Verification items for the finished model (mm, model axes). Round coordinates to 2 decimals unless told otherwise and drop trailing zeros. Loops run counter-clockwise (first coordinate to the right, second up) from the corner with the lowest first, then second, coordinate; pieces in that order, holes last. Notation, with made-up numbers: M 26.5,-38.5 L 63.5,-38.5 A21 cw 63.5,-27.5 Z; hole C -1.5,81.25 d5. An arc over 180 degrees is marked long. Write item = value, one per line. Start each with the question number.
Autodesk Inventor part; units mm, degrees
ref_plane "YZ Plane" through (0, 0, 0) normal (1, 0, 0) x (0, 1, 0)
ref_plane "XZ Plane" through (0, 0, 0) normal (0, 1, 0) x (-1, 0, 0)
ref_plane "XY Plane" through (0, 0, 0) normal (0, 0, 1) x (1, 0, 0)
ref_plane "Work Plane1" through (3, 4, -1) normal (0, 0, 1) x (0, -1, 0)
sketch "Sketch1" plane through (3, 4, -1) normal (0, 0, 1) x (0, -1, 0)
  line L0 (18.0177, 33.5) -> (5, 33.5)
  line L1 (5, 0) -> (5, 33.5)
  line L2 (5, 0) -> (89.75, 0)
  line L3 (89.75, 0) -> (89.75, 33.5)
  line L4 (5, 0) -> (60, 0)
  line L5 (5, -3) -> (5, 0)
  line L6 (4, -3) -> (60, -3)
  line L7 (60, 33.5) -> (60, 3.25)
  line L8 (60, -3) -> (60, 0)
  arc A0 (63.25, 0) -> (60, 3.25) centre (63.25, 3.25) ccw
  line L9 (88.5, 0) -> (183, 0)
  circle A1 centre (75.375, 15.375) radius 6.75
  line L10 (60, 0) -> (60, 33.5)
  circle A2 centre (32.5, 10.5) radius 5.5
  circle A3 centre (9, 4) radius 2.1
  circle A4 centre (9, 29.5) radius 2.1
  circle A5 centre (56.5, 3.5) radius 2.1
  spline S0 degree 2 poles (19.3669, 33.5) (18.6923, 33.3555) (18.0177, 33.5) knots 0 0 0 0.135703 0.135703 0.135703 weights 1 1.02375 1
  line L11 (89.75, 33.5) -> (85.2105, 33.5)
  spline S1 degree 2 poles (85.2105, 33.5) (84.25, 33.2071) (83.2895, 33.5) knots 0 0 0 0.194422 0.194422 0.194422 weights 1 1.05 1
  line L12 (83.2895, 33.5) -> (66.5855, 33.5)
  spline S2 degree 2 poles (66.5855, 33.5) (65.625, 33.2071) (64.6645, 33.5) knots 0 0 0 0.194422 0.194422 0.194422 weights 1 1.05 1
  line L13 (64.6645, 33.5) -> (47.1605, 33.5)
  spline S3 degree 2 poles (47.1605, 33.5) (46.2, 33.2071) (45.2395, 33.5) knots 0 0 0 0.194422 0.194422 0.194422 weights 1 1.05 1
  line L14 (45.2395, 33.5) -> (19.3669, 33.5)
  line L15 (63.25, 0) -> (88.5, 0)
  circle A6 centre (88.5, 3.25) radius 3.25
  line L16 (183, 0) -> (183, 4.5)
  line L17 (183, 4.5) -> (137.8889, 33.5)
  line L18 (137.8889, 33.5) -> (60, 33.5)
  point P0 (52, 0)
  point P1 (64.076, 0)
  point P2 (87.674, 0)
  point P3 (63.25, 3.25)
  point P4 (60, 3.25)
  point P5 (60, 3.25)
extrude "Extrusion1" add sketch "Sketch1" along normal blind 1 contours S0 L14 S3 L13 L7 L10 L2 L1 L0 | A2 | A3 | A4 | A5
sketch "Sketch2" plane through (3, 4, 0) normal (0, 0, 1) x (1, 0, 0)
  line L0 (12.5287, -34.71) -> (8.4496, -34.6899)
  arc A0 (8.4713, -30.29) -> (8.4496, -34.6899) centre (10.5, -32.5) ccw
  line L1 (8.4713, -30.29) -> (12.5504, -30.3101)
  arc A1 (12.5287, -34.71) -> (12.5504, -30.3101) centre (10.5, -32.5) ccw
  circle A2 centre (10.5, -32.5) radius 3
  circle A3 centre (10.5, -32.5) radius 3.5
  point P0 (-3, -4)
  dimension "d5" = 0.5
extrude "Extrusion2" cut sketch "Sketch2" against normal up to next contours A2 L0 | L0 A0 L1 A1 | A2 L1 | A3
sketch "Sketch3" plane through (3, 4, 0) normal (0, 0, 1) x (1, 0, 0)
  circle A0 centre (10.5, -32.5) radius 3.5
  line L0 (0, -5) -> (0, -60)
  line L1 (33.5, -18.0177) -> (33.5, -5)
  line L2 (33.5, -5) -> (0, -5)
  circle A1 centre (3.5, -56.5) radius 3.5
  circle A2 centre (4, -9) radius 4
  circle A3 centre (3.5, -56.5) radius 2.6
  circle A4 centre (4, -9) radius 2.6
  circle A5 centre (29.5, -9) radius 4
  circle A6 centre (29.5, -9) radius 2.6
  line L3 (33.5, -60) -> (33.5, -47.1605)
  line L4 (33.5, -45.2395) -> (33.5, -19.3669)
  line L5 (0, -60) -> (33.5, -60)
  point P0 (-3, -4)
  dimension "d8" = 7
  dimension "d17" = 8
  dimension "d18" = 5.2
  dimension "d19" = 5.2
  dimension "d20" = 4
  dimension "d21" = 4
  dimension "d22" = 8
  dimension "d23" = 5.2
  dimension "d24" = 4
  dimension "d25" = 4
hole "Hole1" at (6.5, -52.5, 0) at (7, -5, 0) at (32.5, -5, 0) direction (0, 0, -1) diameter 3.6 end through all countersink diameter 6.2 countersink angle 90
properties part number "right_metal_gear_bracker"
1. Thickness scan on line 1 (Y direction, x = 13.5, z = -0.45); line 2 (Y direction, x = 7, z = -0.5); line 3 (X direction, y = -30, z = -0.05). Record the ranges inside material, lowest first.
2. Section check C-C, the plane z = -0.7. Give the number of separate pieces and of enclosed holes in the cut face, and give its area (3 significant figures).
3. Mould release check, pull along X, two halves, no side actions. Record for faces 1 (the cylindrical face through (13.04, -25.03, -0.49)), 2 (the flat face through (3, -28.1, -0.5)), 3 (the flat face through (19.5, -1, -0.5)), 4 (the flat face through (36.5, -49.7, -0.5)): pulls with the +X half, pulls with the -X half, needs draft (parallel to the pull), parting line crosses it, or undercut.
4. Section check B-B, the plane x = 13.5. Enter the section's corners in (y, z).
5. Gauge pin test, flat end, axial feed: P1, Ø5, axis at x = 8, y = -46, coming from the +Z side. Record the tip position at first contact, or that the pin passes through.
6. Section check A-A, the plane y = -28.5. Enter the section's corners in (x, z).
Computed values:
q1.line_1 = -56 to -32, -25 to -1
q1.line_2 = -56 to -55.05, -49.95 to -7.6, -2.4 to -1
q1.line_3 = 3 to 10.34, 16.66 to 36.5
q2.separate_pieces = 1
q2.enclosed_holes = 4
q2.area = 1,750 mm2
q3.face_1 = undercut
q3.face_2 = pulls with the -X half
q3.face_3 = needs draft
q3.face_4 = pulls with the +X half
q4.outline = M -56,-1 L -32,-1 L -32,0 L -56,0 Z; M -25,-1 L -1,-1 L -1,0 L -25,0 Z
q5.P1 = 0
q6.outline = M 3,-1 L 10,-1 L 10,0 L 3,0 Z; M 17,-1 L 36.5,-1 L 36.5,0 L 17,0 Z
